Design review of the part built by this model. Coordinates are the model's own, in mm. Coordinates: 2 decimals unless noted, no trailing zeros. Write each loop counter-clockwise with the first axis right and the second up, starting at its lowest first coordinate (ties: lowest second). Pieces come first, ordered by that corner, then holes.
Q1. Add section A-A, the plane z = 5.75. Give the boundary of the cut face in (x, y).
Q2. To check wall thickness, follow probe 1 along X at (y, z) = (-2.5, 4.5); probe 2 along Y at (x, z) = (-38, 5.5); probe 3 along X at (y, z) = (3.25, 1.25). State the ranges of each line that lie inside material, in increasing order.
Q3. Clearance check with a flat-ended pin moving along its axis: pin 1 Ø1.5 at (y, z) = (0.5, 5.5) entering from -X. State where the tip first meets the part, or that it passes through.
Solid Edge part; units mm, degrees
sketch "Sketch1" plane through (10.8674, 10.8674, 0) normal (0, 0, 1) x (1, 0, 0)
  line L0 (-47.8674, -6.8674) -> (-10.8674, -6.8674)
  arc A0 (-10.8674, -6.8674) -> (-10.8674, -14.8674) centre (-10.8674, -10.8674) cw
  line L1 (-10.8674, -14.8674) -> (-47.8674, -14.8674)
  arc A1 (-47.8674, -6.8674) -> (-47.8674, -14.8674) centre (-47.8674, -10.8674) ccw
extrude "Protrusion1" add sketch "Sketch1" along normal blind 7
chamfer "Chamfer_1" distance 0.3 angle 45 8 edges at (-18.5, -4, 7) (-41, 0, 7) (-18.5, 4, 7) (4, 0, 7) (-18.5, -4, 0) (-41, 0, 0) (-18.5, 4, 0) (4, 0, 0)
properties material "Steel"
Here are the results:
1. outline: (-37, -4) - (0, -4) arc R4 ccw to (0, 4) - (-37, 4) arc R4 ccw to start
2. probe 1: x = -40.12 to 3.12
2. probe 2: y = -3.87 to 3.87
2. probe 3: x = -39.33 to 2.33
3. pin 1: stops at x = -41
